Build history of the part. All positions in model axes, mm. A direction names the side the tool comes from. Round coordinates to 2 decimals unless told otherwise and drop trailing zeros. Loops run counter-clockwise (first coordinate to the right, second up) from the corner with the lowest first, then second, coordinate; pieces in that order, holes last. Notation, with made-up numbers: (30.5, 1) - (57.5, 1) arc R20 cw to (57.5, 5) - close; hole circle Ø7 at (-12, 41). An arc over 180 degrees is marked (long way). Answer as CSV lines item,"result". Start each with the question number.
```python
from build123d import *

# Parameters (mm, degrees)
SKETCH2_R           = 10.16
SKETCH2_R_2         = 3.81
BOSS_EXTRUDE1_DEPTH = 1.778
SKETCH2_3_R         = 10.16
SKETCH2_3_R_2       = 3.81
BOSS_EXTRUDE2_DEPTH = 1.778
SKETCH2_4_R         = 3.81
BOSS_EXTRUDE3_DEPTH = 4.572


with BuildPart() as part:
    # Sketch2 → Boss-Extrude1 (new body)
    with BuildSketch(Plane.XY):
        Circle(SKETCH2_R)
        Circle(SKETCH2_R_2, mode=Mode.SUBTRACT)
    extrude(amount=BOSS_EXTRUDE1_DEPTH)

    # Sketch2<3> → Boss-Extrude2 (add)
    with BuildSketch(Plane.XY):
        Circle(SKETCH2_3_R)
        Circle(SKETCH2_3_R_2, mode=Mode.SUBTRACT)
    extrude(amount=BOSS_EXTRUDE2_DEPTH)

    # Sketch2<4> → Boss-Extrude3 (add)
    with BuildSketch(Plane.XY):
        Circle(SKETCH2_4_R)
    extrude(amount=BOSS_EXTRUDE3_DEPTH)


solid = part.part
```
Q1. Band-saw the part on A-A, the plane y = 0. List the corners of the cut face in (x, z).
Q2. Tool access for faces 1 (the flat face through (4, 0, 1.778)), 2 (the cylindrical face through (-1.323, 10.074, 0.877)): list every direction of +Z, -Z, +X, -X, +Y, -Y with a clear straight run to the whole face (end or side of a thin tool).
Q3. Band-saw the part on C-C, the plane z = 1.3. List the corners of the cut face in (x, y), then the cut area to 3 significant figures.
Q4. Band-saw the part on D-D, the plane z = 2.7. List the corners of the cut face in (x, y), then the cut area to 3 significant figures.
Q5. Pin check, flat tip, straight feed: pin 1 Ø3 at (x, y) = (-7.5, -8) entering from +Z. Stop position of the tip, or through.
Q6. Wall check: probe 1 along X at (y, z) = (-0.25, 1.4); probe 2 along Z at (x, y) = (-0.5, 7.5); probe 3 along Y at (x, z) = (0, 2.55). Give the ranges that are in metal, low to high. Write a range as [from, to].
Reported:
1,outline,"(-10.16, 0) - (10.16, 0) - (10.16, 1.78) - (3.81, 1.78) - (3.81, 4.57) - (-3.81, 4.57) - (-3.81, 1.78) - (-10.16, 1.78) - close"
2,face 1,"+Z"
2,face 2,"+Z, -Z"
3,outline,"circle Ø20.32 at (0, 0)"
3,area,"324 mm2"
4,outline,"circle Ø7.62 at (0, 0)"
4,area,"45.6 mm2"
5,pin 1,"stops at z = 1.78"
6,probe 1,"x = [-10.16, 10.16]"
6,probe 2,"z = [0, 1.78]"
6,probe 3,"y = [-3.81, 3.81]"
